```python
from build123d import *

# Parameters (mm, degrees)
SKETCH1_W           = 200
SKETCH1_H           = 90
SKETCH1_R           = 3.25
SKETCH1_R_2         = 40
BOSS_EXTRUDE1_DEPTH = 10
FILLET1_R           = 45
FILLET2_R           = 10


with BuildPart() as part:
    # Sketch1 → Boss-Extrude1 (new body)
    with BuildSketch(Plane.XY):
        with Locations((40.245231608, 0)):
            Rectangle(SKETCH1_W, SKETCH1_H)
        with Locations((-50.110107452, 35.355339059)):
            Circle(SKETCH1_R, mode=Mode.SUBTRACT)
        with Locations((20.600570667, 35.355339059)):
            Circle(SKETCH1_R, mode=Mode.SUBTRACT)
        with Locations((20.600570667, -35.355339059)):
            Circle(SKETCH1_R, mode=Mode.SUBTRACT)
        with Locations((-50.110107452, -35.355339059)):
            Circle(SKETCH1_R, mode=Mode.SUBTRACT)
        with Locations((-14.754768392, 0)):
            Circle(SKETCH1_R_2, mode=Mode.SUBTRACT)
        with Locations((40.245231608, 0)):
            Circle(SKETCH1_R, mode=Mode.SUBTRACT)
        with Locations((70.245231608, 0)):
            Circle(SKETCH1_R, mode=Mode.SUBTRACT)
        with Locations((100.245231608, 0)):
            Circle(SKETCH1_R, mode=Mode.SUBTRACT)
        with Locations((130.245231608, 0)):
            Circle(SKETCH1_R, mode=Mode.SUBTRACT)
    extrude(amount=BOSS_EXTRUDE1_DEPTH)

    # Fillet1
    fillet1_edges = [part.edges().sort_by_distance(p)[0] for p in [
        (140.245231608, -45, 5),
        (140.245231608, 45, 5),
    ]]
    fillet(fillet1_edges, radius=FILLET1_R - 0.0001)  # a hair under: the kernel refuses the full size

    # Fillet2
    fillet2_edges = [part.edges().sort_by_distance(p)[0] for p in [
        (-59.754768392, -45, 5),
        (-59.754768392, 45, 5),
    ]]
    fillet(fillet2_edges, radius=FILLET2_R)


solid = part.part
```
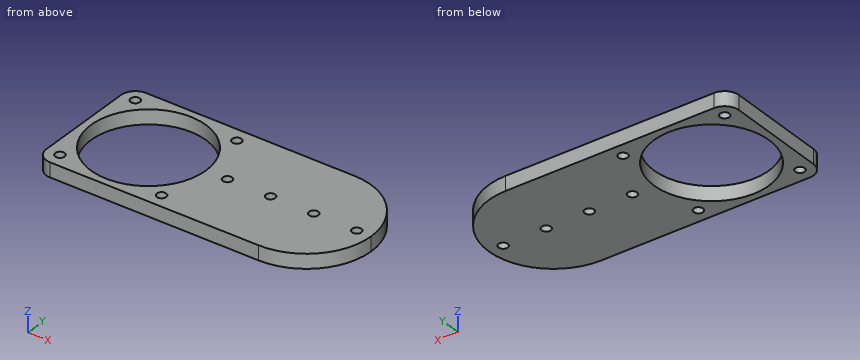
CAD build for the part. Positions are in the model's coordinates, mm. Round coordinates to 2 decimals unless told otherwise and drop trailing zeros. Order: outer loops, then holes, each group sorted by start corner. A loop starts at its lowest first (then second) coordinate and runs counter-clockwise, first axis right, second up. Notation, with made-up numbers: (36.25, -22.75) -> (43.25, -22.75) arc R6 cw to (43.25, -11.75) -> close; hole circle Ø11 at (12, 31). An arc over 180 degrees is marked (long way). One line per question, with ' | ' between items.
Q1. Probe probe 1 along X at (y, z) = (-1.5, 1.75); probe 2 along X at (y, z) = (25, 9.75); probe 3 along Y at (x, z) = (-27, 1.75). List the from-to ranges inside material, lowest first.
Completed:
probe 1: x = -59.75 to -54.73, 25.22 to 37.36, 43.13 to 67.36, 73.13 to 97.36, 103.13 to 127.36, 133.13 to 140.22 | probe 2: x = -59.75 to -45.98, 16.47 to 132.66 | probe 3: y = -45 to -38.08, 38.08 to 45
Q2. Slice it at B-B (x = 10). Write the cut outline in (y, z).
Completed:
outline: (-45, 0) -> (-31.42, 0) -> (-31.42, 10) -> (-45, 10) -> close; (31.42, 0) -> (45, 0) -> (45, 10) -> (31.42, 10) -> close
Q3. Slice it at A-A (y = 10). Write the cut outline in (x, z).
Completed:
outline: (-59.75, 0) -> (-53.48, 0) -> (-53.48, 10) -> (-59.75, 10) -> close; (23.98, 0) -> (139.12, 0) -> (139.12, 10) -> (23.98, 10) -> close
Q4. Drop flat-ended pins along their axis: pin 1 (1 mm diameter, centred on y = -31, z = 5.5, fed in from +X); pin 2 (4 mm diameter, centred on x = -50.11, y = -35.36, fed in from -Z); pin 3 (3 mm diameter, centred on y = 20.5, z = 4.5, fed in from +X). Give the stop position or say it passes through.
Completed:
pin 1: stops at x = 128.33 | pin 2: passes through | pin 3: stops at x = 136.04
Q5. Slice it at C-C (z = 6.5). Give the number of separate pieces and of enclosed holes in the cut face, then the cut area to 3 significant figures.
Completed:
separate pieces: 1 | enclosed holes: 9 | area: 11,800 mm^2
